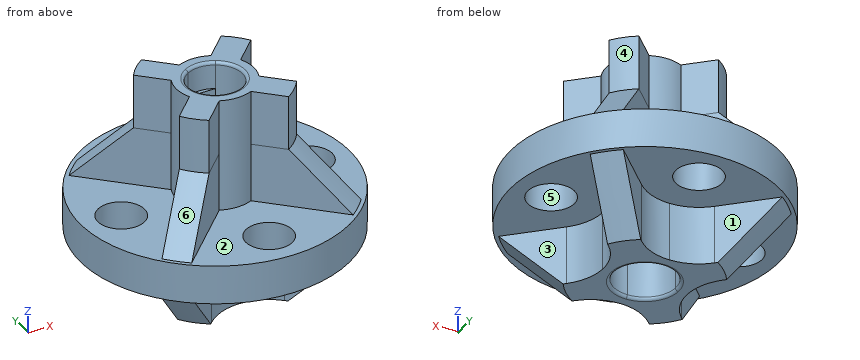
from build123d import *
from build123d.topology import SkipClean

# Parameters (mm, degrees)
SKETCH2_R           = 33.6
SKETCH2_R_2         = 2
SKETCH2_R_3         = 6
BOSS_EXTRUDE1_DEPTH = 10
BOSS_EXTRUDE2_START = 15
BOSS_EXTRUDE2_DEPTH = 15
CIRPATTERN1_COUNT   = 4
SKETCH4_R           = 10
BOSS_EXTRUDE3_DEPTH = 29
SKETCH5_R           = 34.6
SKETCH5_R_2         = 33.6
BOSS_EXTRUDE5_DEPTH = 10
BOSS_EXTRUDE6_START = 4
SKETCH6_R           = 8
SKETCH6_R_2         = 2
BOSS_EXTRUDE6_DEPTH = 4
BOSS_EXTRUDE7_DEPTH = 15
CIRPATTERN2_COUNT   = 4
CHAMFER1_SIZE       = 15
CHAMFER2_SIZE       = 15
BOSS_EXTRUDE8_DEPTH = 14
CUT_EXTRUDE1_START  = -7
SKETCH10_R          = 7.05
CUT_EXTRUDE1_DEPTH  = 7
FILLET1_R           = 0.75


with BuildPart() as part:
    # Sketch2 → Boss-Extrude1 (new body)
    with BuildSketch(Plane.XY):
        Circle(SKETCH2_R)
        Circle(SKETCH2_R_2, mode=Mode.SUBTRACT)
        with Locations((0, 24.6)):
            Circle(SKETCH2_R_3, mode=Mode.SUBTRACT)
        with Locations((0, -24.6)):
            Circle(SKETCH2_R_3, mode=Mode.SUBTRACT)
        with Locations((-24.6, 0)):
            Circle(SKETCH2_R_3, mode=Mode.SUBTRACT)
        with Locations((24.6, 0)):
            Circle(SKETCH2_R_3, mode=Mode.SUBTRACT)
    extrude(amount=BOSS_EXTRUDE1_DEPTH)

    # Sketch3 → Boss-Extrude2 (add)
    with BuildSketch(Plane(origin=(0, 0, 0), x_dir=(-1, 0, 0), z_dir=(0, 0, -1)).offset(BOSS_EXTRUDE2_START)):
        with BuildLine():
            Line((-8, 0), (-11.1, 0))
            ThreePointArc((-11.1, 0), (-12.127626311, -5.166226337), (-15.054058454, -9.545941546))
            Line((-15.054058454, -9.545941546), (-26.352684728, -20.84456782))
            ThreePointArc((-26.352684728, -20.84456782), (-23.758787848, -23.758787848), (-20.84456782, -26.352684728))
            Line((-20.84456782, -26.352684728), (-9.545941546, -15.054058454))
            ThreePointArc((-9.545941546, -15.054058454), (-5.166226337, -12.127626311), (0, -11.1))
            Line((0, -11.1), (0, -8))
            ThreePointArc((0, -8), (-5.656854249, -5.656854249), (-8, 0))
        make_face()
    boss_extrude2 = extrude(amount=-BOSS_EXTRUDE2_DEPTH)

    # CirPattern1: Boss-Extrude2 ×4 about axis
    with SkipClean():  # the faces are left unmerged after this step: merging them gives an invalid solid
        cirpattern1_axis = Axis((0, 0, 0), (0, 0, 1))
        for i in range(1, CIRPATTERN1_COUNT):
            add(boss_extrude2.rotate(cirpattern1_axis, i * 360 / CIRPATTERN1_COUNT))

    # Sketch4 → Boss-Extrude3 (add)
    with SkipClean():  # the faces are left unmerged after this step: merging them gives an invalid solid
        with BuildSketch(Plane.XY.offset(10)):
            with Locations(Location((0, 0, 0), (0, 0, 180))):
                Circle(SKETCH4_R)
            with BuildLine():
                Line((-3.619392214, 6.05), (3.619392214, 6.05))
                ThreePointArc((3.619392214, 6.05), (0, -7.05), (-3.619392214, 6.05))
            make_face(mode=Mode.SUBTRACT)
        extrude(amount=BOSS_EXTRUDE3_DEPTH)

    # Sketch5 → Boss-Extrude5 (add)
    with BuildSketch(Plane(origin=(0, 0, 0), x_dir=(-1, 0, 0), z_dir=(0, 0, -1))):
        Circle(SKETCH5_R)
        Circle(SKETCH5_R_2, mode=Mode.SUBTRACT)
    extrude(amount=-BOSS_EXTRUDE5_DEPTH)

    # Sketch6 → Boss-Extrude6 (add)
    with SkipClean():  # the faces are left unmerged after this step: merging them gives an invalid solid
        with BuildSketch(Plane(origin=(0, 0, 0), x_dir=(-1, 0, 0), z_dir=(0, 0, -1)).offset(BOSS_EXTRUDE6_START)):
            with Locations(Location((0, 0, 0), (0, 0, 180))):
                Circle(SKETCH6_R)
            Circle(SKETCH6_R_2, mode=Mode.SUBTRACT)
        extrude(amount=-BOSS_EXTRUDE6_DEPTH)

    # Sketch8 → Boss-Extrude7 (add)
    with SkipClean():  # the faces are left unmerged after this step: merging them gives an invalid solid
        with BuildSketch(Plane.XY.offset(10)):
            with BuildLine():
                Line((21.154662867, -26.104410336), (4.148946916, -9.098694384))
                ThreePointArc((4.148946916, -9.098694384), (7.071067812, -7.071067812), (9.098694384, -4.148946916))
                Line((9.098694384, -4.148946916), (26.104410336, -21.154662867))
                ThreePointArc((26.104410336, -21.154662867), (23.758787848, -23.758787848), (21.154662867, -26.104410336))
            make_face()
        boss_extrude7 = extrude(amount=BOSS_EXTRUDE7_DEPTH)

    # CirPattern2: Boss-Extrude7 ×4 about axis
    with SkipClean():  # the faces are left unmerged after this step: merging them gives an invalid solid
        cirpattern2_axis = Axis((0, 0, 0), (0, 0, 1))
        for i in range(1, CIRPATTERN2_COUNT):
            add(boss_extrude7.rotate(cirpattern2_axis, i * 360 / CIRPATTERN2_COUNT))

    # Chamfer1
    chamfer1_edges = [part.edges().sort_by_distance(p)[0] for p in [
        (23.758787848, 23.758787848, -15),
        (23.758787848, -23.758787848, -15),
        (-23.758787848, -23.758787848, -15),
        (-23.758787848, 23.758787848, -15),
    ]]
    chamfer(chamfer1_edges, length=CHAMFER1_SIZE - 0.0001)  # a hair under: the kernel refuses the full size

    # Chamfer2
    chamfer2_edges = [part.edges().sort_by_distance(p)[0] for p in [
        (23.758787848, -23.758787848, 25),
        (-23.758787848, -23.758787848, 25),
        (-23.758787848, 23.758787848, 25),
        (23.758787848, 23.758787848, 25),
    ]]
    chamfer(chamfer2_edges, length=CHAMFER2_SIZE - 0.0001)  # a hair under: the kernel refuses the full size

    # Sketch9 → Boss-Extrude8 (add)
    with BuildSketch(Plane.XY.offset(25)):
        with BuildLine():
            Line((4.148946916, 9.098694384), (10.442362812, 15.392110281))
            ThreePointArc((10.442362812, 15.392110281), (13.15218613, 13.15218613), (15.392110281, 10.442362812))
            Line((15.392110281, 10.442362812), (9.098694384, 4.148946916))
            ThreePointArc((9.098694384, 4.148946916), (7.071067812, 7.071067812), (4.148946916, 9.098694384))
        make_face()
        with BuildLine():
            Line((10.442362812, -15.392110281), (4.148946916, -9.098694384))
            ThreePointArc((4.148946916, -9.098694384), (7.071067812, -7.071067812), (9.098694384, -4.148946916))
            Line((9.098694384, -4.148946916), (15.392110281, -10.442362812))
            ThreePointArc((15.392110281, -10.442362812), (13.15218613, -13.15218613), (10.442362812, -15.392110281))
        make_face()
        with BuildLine():
            Line((-15.392110281, -10.442362812), (-9.098694384, -4.148946916))
            ThreePointArc((-9.098694384, -4.148946916), (-7.071067812, -7.071067812), (-4.148946916, -9.098694384))
            Line((-4.148946916, -9.098694384), (-10.442362812, -15.392110281))
            ThreePointArc((-10.442362812, -15.392110281), (-13.15218613, -13.15218613), (-15.392110281, -10.442362812))
        make_face()
        with BuildLine():
            Line((-15.392110281, 10.442362812), (-9.098694384, 4.148946916))
            ThreePointArc((-9.098694384, 4.148946916), (-7.071067812, 7.071067812), (-4.148946916, 9.098694384))
            Line((-4.148946916, 9.098694384), (-10.442362812, 15.392110281))
            ThreePointArc((-10.442362812, 15.392110281), (-13.15218613, 13.15218613), (-15.392110281, 10.442362812))
        make_face()
    extrude(amount=BOSS_EXTRUDE8_DEPTH)

    # Sketch10 → Cut-Extrude1 (cut)
    with SkipClean():  # the faces are left unmerged after this step: merging them gives an invalid solid
        with BuildSketch(Plane.XY.offset(39).offset(CUT_EXTRUDE1_START)):
            with Locations(Location((0, 0, 0), (0, 0, 120.889831942))):
                Circle(SKETCH10_R)
        extrude(amount=CUT_EXTRUDE1_DEPTH, mode=Mode.SUBTRACT)

    # Fillet1
    fillet1_edges = [part.edges().sort_by_distance(p)[0] for p in [
        (8, 0, -15),
        (0, -7.05, 39),
    ]]
    fillet(fillet1_edges, radius=FILLET1_R)


solid = part.part
For this review, take the finished solid that the model builds, in its own axes (mm). Face numbers are marked on the shaded views. A direction names the side the tool comes from. Coordinates: 2 decimals unless noted, no trailing zeros. Order: outer loops, then holes, each group sorted by start corner. A loop starts at its lowest first (then second) coordinate and runs counter-clockwise, first axis right, second up. Notation, with made-up numbers: (36, 82) -> (59, 82) arc R23 ccw to (59, 99) -> close; hole circle Ø2 at (32.25, -36.5). An arc over 180 degrees is marked (long way). Return JSON: item names as keys, results as strings.
1. For pin 1 Ø1.5 at (x, y) = (23.5, -18) entering from -Z; pin 2 Ø1.5 at (x, y) = (27.5, -11.5) entering from -Z; pin 3 Ø1 at (x, y) = (-2.5, -6) entering from +Z; pin 4 Ø10 at (y, z) = (-24, 24.5) entering from -X, all flat-tipped, find the tip position at first contact; note any pin that passes through.
Answer block:
{"pin 1": "z = -4.75", "pin 2": "z = 0", "pin 3": "z = 10", "pin 4": "through"}
2. We need section A-A on z = 28. Write out the cut boundary in (x, y), and give its area (3 significant figures).
Answer block:
{"outline": "(-15.39, -10.44) arc R18.6 ccw to (-10.44, -15.39) -> (-4.15, -9.1) arc R10 ccw to (4.15, -9.1) -> (10.44, -15.39) arc R18.6 ccw to (15.39, -10.44) -> (9.1, -4.15) arc R10 ccw to (9.1, 4.15) -> (15.39, 10.44) arc R18.6 ccw to (10.44, 15.39) -> (4.15, 9.1) arc R10 ccw to (-4.15, 9.1) -> (-10.44, 15.39) arc R18.6 ccw to (-15.39, 10.44) -> (-9.1, 4.15) arc R10 ccw to (-9.1, -4.15) -> close; hole (-3.62, 6.05) arc R7.05 ccw (long way) to (3.62, 6.05) -> close", "area": "406 mm²"}
3. We need section C-C on x = 29.5. Write out the cut boundary in (y, z), and give its area (3 significant figures).
Answer block:
{"outline": "(-18.08, 0) -> (-3.46, 0) -> (-3.46, 10) -> (-18.08, 10) -> close; (3.46, 0) -> (18.08, 0) -> (18.08, 10) -> (3.46, 10) -> close", "area": "292 mm²"}
4. The part is to be moulded in two halves that separate along X. For the marked faces 4, 5 and 6, say which applies: +X half, -X half, draft (parallel to the pull), parting line (faces both ways), or undercut.
Answer block:
{"face 4": "+X half", "face 5": "undercut", "face 6": "-X half"}
5. For line 1 (Y direction, x = 0, z = 7.5); line 2 (Y direction, x = 0, z = 26); line 3 (X direction, y = 0.5, z = 17.5), list the stretches that pass through material, from the lowest coordinate up. Write a range as from..to.
Answer block:
{"line 1": "-34.6..-30.6, -18.6..-2, 2..18.6, 30.6..34.6", "line 2": "-10..-7.05, 6.05..10", "line 3": "-9.99..-7.03, 7.03..9.99"}
6. We need section B-B on y = -28. Write out the cut boundary in (x, z).
Answer block:
{"outline": "(-20.33, 0) -> (-4.94, 0) -> (-4.94, 10) -> (-20.33, 10) -> close; (4.94, 0) -> (20.33, 0) -> (20.33, 10) -> (4.94, 10) -> close"}
7. Machinability: for the marked faces 1, 2 and 3, which of the approach directions +Z, -Z, +X, -X, +Y, -Y give a long, thin tool a straight path to every point of the face, cutting with its end or side? Answer none if there is none.
Answer block:
{"face 1": "-Z, +Y", "face 2": "+Z", "face 3": "-Z, +X"}
8. We need section D-D on z = 5. Write out the cut boundary in (x, y).
Answer block:
{"outline": "circle Ø69.2 at (0, 0); hole circle Ø12 at (-24.6, 0); hole circle Ø12 at (0, -24.6); hole circle Ø12 at (0, 24.6); hole circle Ø4 at (0, 0); hole circle Ø12 at (24.6, 0)"}
